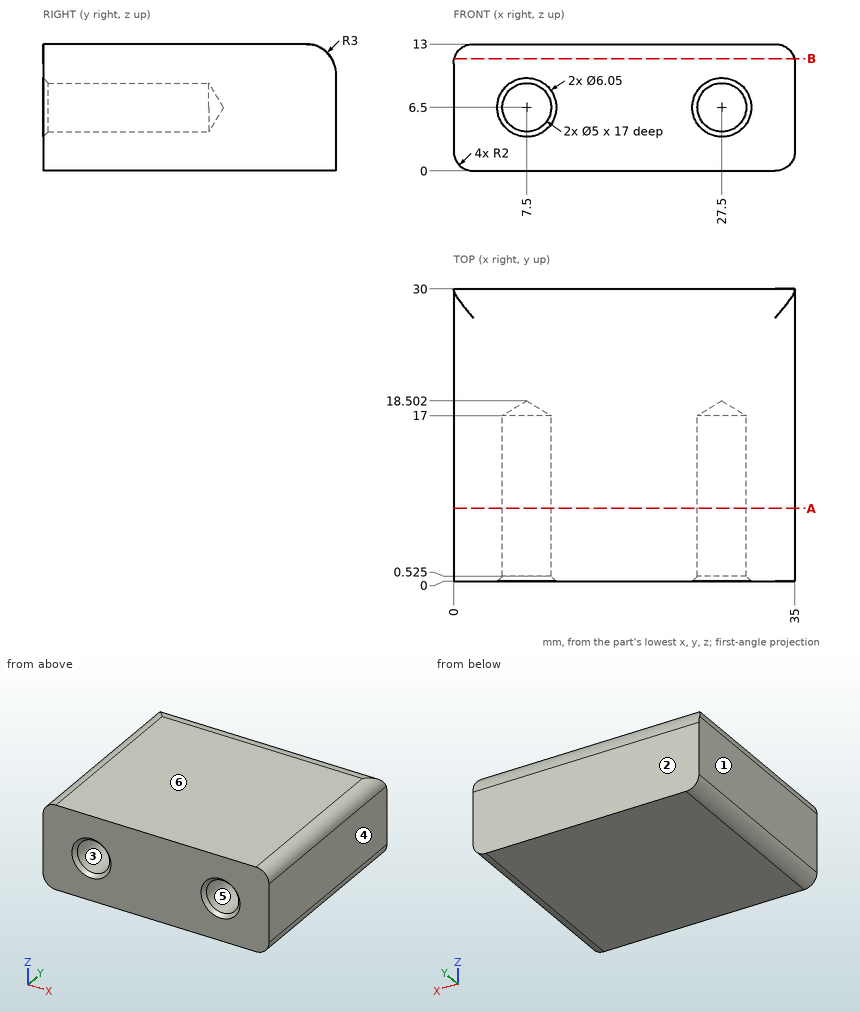
Design review of the part shown in the three views and the two pictorial views. Dimensions are in mm from the part's minimum x, y and z. A direction names the side the tool comes from. Round coordinates to 2 decimals unless told otherwise and drop trailing zeros. Loops run counter-clockwise (first coordinate to the right, second up) from the corner with the lowest first, then second, coordinate; pieces in that order, holes last. Notation, with made-up numbers: M -29.75,-24.5 L -7.75,-24.5 A14 ccw -7.75,-3.5 Z; hole C 60.25,65 d1. An arc over 180 degrees is marked long. Answer as a JSON object with one key per item and string values.
Item 1: We need section B-B, the plane z = 11.5. State the section outline as (x, y) points.
Check sheet entries:
{"outline": "M 0.06,0 L 34.94,0 L 34.94,29.6 L 0.06,29.6 Z"}
Item 2: Clearance check with a flat-ended pin moving along its axis: P1, Ø6, axis at x = 27.5, z = 6.5, coming from the -Y side (1 decimal). State where the tip first meets the part, or that it passes through.
Check sheet entries:
{"P1": "y = 0"}
Item 3: We need section A-A, the plane y = 7.5. State the section outline as (x, z) points, and give its area (3 significant figures).
Check sheet entries:
{"outline": "M 0,2 A2 ccw 2,0 L 33,0 A2 ccw 35,2 L 35,11 A2 ccw 33,13 L 2,13 A2 ccw 0,11 Z; hole C 7.5,6.5 d5; hole C 27.5,6.5 d5", "area": "412 mm2"}
Item 4: For line 1 along Z through (x, y) = (7.5, 7.5); line 2 along Z through (x, y) = (27, 13); line 3 along X through (y, z) = (16.5, 7), list the stretches that pass through material, from the lowest coordinate up.
Check sheet entries:
{"line 1": "0 to 4, 9 to 13", "line 2": "0 to 4.05, 8.95 to 13", "line 3": "0 to 5.05, 9.95 to 25.05, 29.95 to 35"}
Item 5: Tool access review of the marked faces 5 and 6: name each direction out of +Z, -Z, +X, -X, +Y, -Y from which nothing blocks a thin tool from reaching the whole face with its end or side.
Check sheet entries:
{"face 5": "-Y", "face 6": "+Z, +X, -X, +Y, -Y"}
Item 6: The part is to be moulded in two halves that separate along X. For the marked faces 1, 2, 3 and 4, say which applies: +X half, -X half, draft (parallel to the pull), parting line (faces both ways), or undercut.
Check sheet entries:
{"face 1": "-X half", "face 2": "draft", "face 3": "undercut", "face 4": "+X half"}
